For this review, take the finished solid that the model builds, in its own axes (mm). Coordinates: 2 decimals unless noted, no trailing zeros. Loops run counter-clockwise (first coordinate to the right, second up) from the corner with the lowest first, then second, coordinate; pieces in that order, holes last. Notation, with made-up numbers: M -19,65.25 L -1,65.25 A27 cw -1,91.25 Z; hole C -6,-27.75 d4. An arc over 180 degrees is marked long. Use one line per item in the form item = value.
```python
from build123d import *

# Parameters (mm, degrees)
F0_W     = 112
F0_H     = 26
F0_R     = 11
F0_W_2   = 54
F0_H_2   = 16
F1_DEPTH = 2


with BuildPart() as f1:
    # F0 (on Top) → F1 (new body)
    with BuildSketch(Plane.XY):
        Rectangle(F0_W, F0_H)
        with Locations((-42, 0)):
            Circle(F0_R, mode=Mode.SUBTRACT)
        Rectangle(F0_W_2, F0_H_2, mode=Mode.SUBTRACT)
        with Locations((42, 0)):
            Circle(F0_R, mode=Mode.SUBTRACT)
    extrude(amount=F1_DEPTH)


solid = f1.part
```
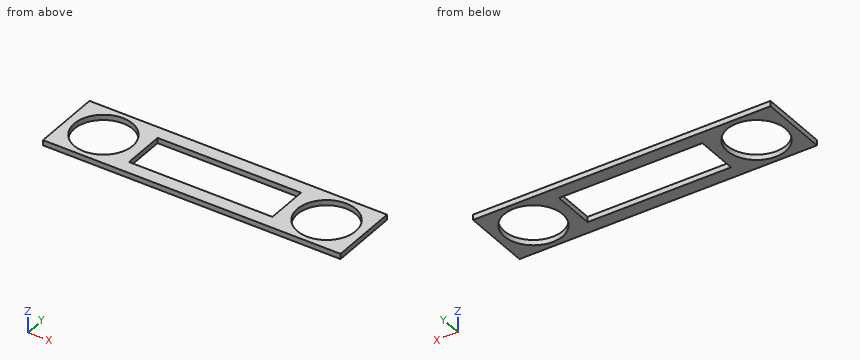
1. Consider section A-A on x = 42. Write out the cut boundary in (y, z).
Computed values:
outline = M -13,0 L -11,0 L -11,2 L -13,2 Z; M 11,0 L 13,0 L 13,2 L 11,2 Z
2. Consider section D-D on y = -9.5. Write out the cut boundary in (x, z).
Computed values:
outline = M -56,0 L -47.55,0 L -47.55,2 L -56,2 Z; M -36.45,0 L 36.45,0 L 36.45,2 L -36.45,2 Z; M 47.55,0 L 56,0 L 56,2 L 47.55,2 Z
3. Consider section B-B on y = 0. Write out the cut boundary in (x, z).
Computed values:
outline = M -56,0 L -53,0 L -53,2 L -56,2 Z; M -31,0 L -27,0 L -27,2 L -31,2 Z; M 27,0 L 31,0 L 31,2 L 27,2 Z; M 53,0 L 56,0 L 56,2 L 53,2 Z
4. Wall thickness on line 1 along X through (y, z) = (-0.25, 0.8); line 2 along Y through (x, z) = (42, 0.6); line 3 along X through (y, z) = (-7, 1.8): over which ranges is each line inside the solid? List them lowest first. Write a range as from..to.
Computed values:
line_1 = -56..-53, -31..-27, 27..31, 53..56
line_2 = -13..-11, 11..13
line_3 = -56..-50.49, -33.51..-27, 27..33.51, 50.49..56
5. Consider section C-C on z = 0.6. Write out the cut boundary in (x, y), plus the area to 3 significant figures.
Computed values:
outline = M -56,-13 L 56,-13 L 56,13 L -56,13 Z; hole C -42,0 d22; hole M -27,-8 L 27,-8 L 27,8 L -27,8 Z; hole C 42,0 d22
area = 1,290 mm2
